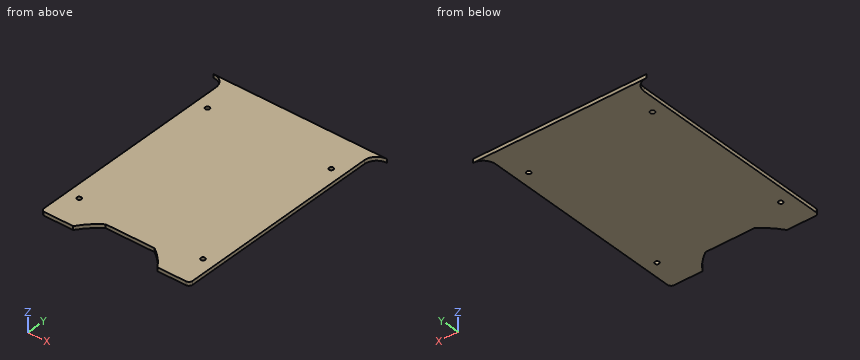
```python
from build123d import *

# Parameters (mm, degrees)
SKETCH1_R           = 1.75
BOSS_EXTRUDE1_DEPTH = 3


with BuildPart() as part:
    # Sketch1 → Boss-Extrude1 (new body)
    with BuildSketch(Plane.XY):
        with BuildLine():
            Line((-70, 219), (70, 219))
            ThreePointArc((70, 219), (62.928932188, 216.071067812), (60, 209))
            Line((60, 209), (60, 42.746292529))
            ThreePointArc((60, 42.746292529), (59.121320344, 40.624972186), (57, 39.746292529))
            Line((57, 39.746292529), (34.010726171, 39.746292529))
            add(Edge.make_bspline(
                [(19.726580418, 54.15), (28.313482158, 48.285383086), (34.010726171, 39.746292529)],
                knots=[0, 0, 0, 1, 1, 1], degree=2))
            Line((19.726580418, 54.15), (-19.726580418, 54.15))
            add(Edge.make_bspline(
                [(-34.01072617, 39.746292529), (-28.313482158, 48.285383086), (-19.726580418, 54.15)],
                knots=[0, 0, 0, 1, 1, 1], degree=2))
            Line((-34.01072617, 39.746292529), (-57, 39.746292529))
            ThreePointArc((-57, 39.746292529), (-59.121320344, 40.624972186), (-60, 42.746292529))
            Line((-60, 42.746292529), (-60, 209))
            ThreePointArc((-60, 209), (-62.928932188, 216.071067812), (-70, 219))
        make_face()
        with Locations((50, 64.746292529)):
            Circle(SKETCH1_R, mode=Mode.SUBTRACT)
        with Locations((50, 189)):
            Circle(SKETCH1_R, mode=Mode.SUBTRACT)
        with Locations((-50, 189)):
            Circle(SKETCH1_R, mode=Mode.SUBTRACT)
        with Locations((-50, 64.746292529)):
            Circle(SKETCH1_R, mode=Mode.SUBTRACT)
    extrude(amount=BOSS_EXTRUDE1_DEPTH)


solid = part.part
```
Here's how the part is built. I have some questions about the finished solid (model axes, mm). Coordinates: 2 decimals unless noted, no trailing zeros. Order: outer loops, then holes, each group sorted by start corner. A loop starts at its lowest first (then second) coordinate and runs counter-clockwise, first axis right, second up.
1) Imagine slicing it at B-B on x = -7. List the corners of the cut face in (y, z) for me, and give its area (3 significant figures).
2) I need wall thicknesses on line 1 (Y direction, x = 50, z = 1.95); line 2 (Y direction, x = -51.5, z = 1.1); line 3 (X direction, y = 170.5, z = 0.4). Which ranges of each line are inside material? Lowest first, please.
3) Will this pin go through, and if not, where does the flat tip stop? pin 1 (0.9 mm diameter, centred on y = 137, z = 1.5, fed in from +X).
4) Imagine slicing it at C-C on z = 2.4. State how many separate pieces and enclosed holes the cut face has, and give its area (3 significant figures).
5) Imagine slicing it at A-A on y = 158. List the corners of the cut face in (x, z) for me, and give its area (3 significant figures).
Response values:
1. outline: (54.15, 0) - (219, 0) - (219, 3) - (54.15, 3) - close
1. area: 495 mm2
2. line 1: y = 39.75 to 63, 66.5 to 187.25, 190.75 to 219
2. line 2: y = 39.75 to 63.84, 65.65 to 188.1, 189.9 to 219
2. line 3: x = -60 to 60
3. pin 1: stops at x = 60
4. separate pieces: 1
4. enclosed holes: 4
4. area: 20,700 mm2
5. outline: (-60, 0) - (60, 0) - (60, 3) - (-60, 3) - close
5. area: 360 mm2
